```python
from build123d import *

# Parameters (mm, degrees)
L_BASE_DEPTH                                = 12.7
SKETCH3_W                                   = 44.45
SKETCH3_H                                   = 25.4
RECTANGULAR_EXTRUDE_DEPTH                   = 10.5664
SKETCH4_W                                   = 11.1125
SKETCH4_H                                   = 25.4
FORK_EXTRUDE_DEPTH                          = 29.3624
SKETCH6_W                                   = 38.1
SKETCH6_H                                   = 3.175
F_4_EXPANSION_INSERT_RECESSES_1_D           = 3.2639
F_4_EXPANSION_INSERT_RECESSES_1_DEPTH       = 19.05
F_4_EXPANSION_INSERT_RECESSES_1_CBORE_D     = 3.96875
F_4_EXPANSION_INSERT_RECESSES_1_CBORE_DEPTH = 4.7625
F_4_EXPANSION_INSERT_RECESSES_1_TIP         = 0.980574487
F_4_EXPANSION_INSERT_RECESSES_2_D           = 3.2639
F_4_EXPANSION_INSERT_RECESSES_2_DEPTH       = 9.525
F_4_EXPANSION_INSERT_RECESSES_2_CBORE_D     = 3.96875
F_4_EXPANSION_INSERT_RECESSES_2_CBORE_DEPTH = 4.7625
F_4_EXPANSION_INSERT_RECESSES_2_TIP         = 0.980574487


with BuildPart() as part:
    # Sketch1 → L-Base (new body)
    with BuildSketch(Plane(origin=(0, 0, 0), x_dir=(1, 0, 0), z_dir=(0, 1, 0))):
        Polygon((0, 0), (44.45, 0), (44.45, 25.4), (20.066, 25.4), (20.066, 39.116), (0, 39.116), align=None)
    extrude(amount=L_BASE_DEPTH)

    # Sketch3 → Rectangular Extrude (add)
    with BuildSketch(Plane(origin=(0, 12.7, 0), x_dir=(1, 0, 0), z_dir=(0, 1, 0))):
        with Locations((22.225, 12.7)):
            Rectangle(SKETCH3_W, SKETCH3_H)
    extrude(amount=RECTANGULAR_EXTRUDE_DEPTH)

    # Sketch4 → Fork Extrude (add)
    with BuildSketch(Plane(origin=(0, 23.2664, 0), x_dir=(1, 0, 0), z_dir=(0, 1, 0))):
        with Locations((5.55625, 12.7)):
            Rectangle(SKETCH4_W, SKETCH4_H)
        with Locations((38.89375, 12.7)):
            Rectangle(SKETCH4_W, SKETCH4_H)
    extrude(amount=FORK_EXTRUDE_DEPTH)

    # Sketch6 → Shaft Recess (revolve, cut)
    with BuildSketch(Plane(origin=(0, 52.6288, 0), x_dir=(1, 0, 0), z_dir=(0, 1, 0))):
        with Locations((22.225, 11.1125)):
            Rectangle(SKETCH6_W, SKETCH6_H)
    revolve(axis=Axis((0, 52.6288, -12.7), (1, 0, 0)), mode=Mode.SUBTRACT)

    # #4 Expansion Insert Recesses #1
    with Locations(Plane(origin=(0, 52.6288, 0), x_dir=(1, 0, 0), z_dir=(0, 1, 0))):
        with Locations((5.55625, 20.6375), (5.55625, 4.7625), (38.89375, 20.6375), (38.89375, 4.7625)):
            CounterBoreHole(F_4_EXPANSION_INSERT_RECESSES_1_D / 2, F_4_EXPANSION_INSERT_RECESSES_1_CBORE_D / 2, F_4_EXPANSION_INSERT_RECESSES_1_CBORE_DEPTH, depth=F_4_EXPANSION_INSERT_RECESSES_1_DEPTH)
            with Locations((0, 0, -(F_4_EXPANSION_INSERT_RECESSES_1_DEPTH + F_4_EXPANSION_INSERT_RECESSES_1_TIP / 2))):  # 118° drill point
                Cone(0, F_4_EXPANSION_INSERT_RECESSES_1_D / 2, F_4_EXPANSION_INSERT_RECESSES_1_TIP, mode=Mode.SUBTRACT)

    # #4 Expansion Insert Recesses #2
    with Locations(Plane(origin=(0, 0, 0), x_dir=(-1, 0, 0), z_dir=(0, -1, 0))):
        with Locations((-10.033, 10.033), (-29.083, 10.033), (-10.033, 29.083)):
            CounterBoreHole(F_4_EXPANSION_INSERT_RECESSES_2_D / 2, F_4_EXPANSION_INSERT_RECESSES_2_CBORE_D / 2, F_4_EXPANSION_INSERT_RECESSES_2_CBORE_DEPTH, depth=F_4_EXPANSION_INSERT_RECESSES_2_DEPTH)
            with Locations((0, 0, -(F_4_EXPANSION_INSERT_RECESSES_2_DEPTH + F_4_EXPANSION_INSERT_RECESSES_2_TIP / 2))):  # 118° drill point
                Cone(0, F_4_EXPANSION_INSERT_RECESSES_2_D / 2, F_4_EXPANSION_INSERT_RECESSES_2_TIP, mode=Mode.SUBTRACT)


solid = part.part
```
Work out the finished part from the listing and answer in its coordinate system (mm). A direction names the side the tool comes from. Give positions to 0.01 mm unless a question says otherwise; leave off trailing zeros. Loops run counter-clockwise (first coordinate to the right, second up) from the corner with the lowest first, then second, coordinate; pieces in that order, holes last. Notation, with made-up numbers: (-24.75, 48.5) -> (-13.75, 48.5) arc R21 cw to (-13.75, 81.5) -> close; hole circle Ø1 at (-11.75, 7.25). An arc over 180 degrees is marked (long way). One line per question, with ' | ' between items. Start each with the question number.
1) For faces 5 (the face through (41.275, 51, -13)), 6 (the face through (33.338, 38, -13)), 7 (the face through (30.64, 7.18, -10.52)), 8 (the face through (22, 0, -15)), determine the directions among +Z, -Z, +X, -X, +Y, -Y from which every point of the face is accessible in a straight line to the end or side of a thin tool.
2) Determine the mould class of faces 1 (the face through (38.86, 32.77, -20.92)), 2 (the face through (37.362, 49.455, -12.63)), 3 (the face through (22, 20, -25.4)), 4 (the face through (0, 26, -15)) for opening direction X: +X half, -X half, draft (parallel to the pull), parting line (faces both ways), or undercut.
3) Section C-C, the plane x = 34 is taken. Determine the outline of the cut face in (y, z) (3 decimals).
4) Straight lines are drawn through the part: L1, parallel to X at y = 25.5, z = -24; L2, parallel to Z at x = 19, y = 13.5; L3, parallel to Y at x = 32, z = -19.5. For each, find the intervals that lie inside material, in ascending order.
5) Section A-A, the plane y = 44.5 is taken. Determine the outline of the cut face in (x, z).
6) Section B-B, the plane y = 27.5 is taken. Determine the outline of the cut face in (x, z), then the cut area to 3 significant figures.
7) Each of these flat-tipped pins is pushed along its axis until it touches: pin 1 (2 mm diameter, centred on x = 39, z = -4, fed in from +Y); pin 2 (1.2 mm diameter, centred on x = 9.5, z = -28, fed in from -Y); pin 3 (4 mm diameter, centred on x = 10.033, z = -29.083, fed in from +Y). Where does it stop, or does it pass through?
Resolved:
1) face 5: +Y | face 6: +Z, -Z, +Y | face 7: -Y | face 8: +Z, -Z, +X, -X, -Y
2) face 1: undercut | face 2: undercut | face 3: draft | face 4: -X half
3) outline: (0, -25.4) -> (52.629, -25.4) -> (52.629, -15.875) arc R3.175 cw to (52.629, -9.525) -> (52.629, 0) -> (0, 0) -> close
4) L1: 0 to 11.11, 33.34 to 44.45 | L2: -25.4 to 0 | L3: 0 to 23.27
5) outline: (0, -25.4) -> (11.11, -25.4) -> (11.11, 0) -> (0, 0) -> close; (33.34, -25.4) -> (44.45, -25.4) -> (44.45, 0) -> (33.34, 0) -> close; hole circle Ø3.26 at (5.56, -20.64); hole circle Ø3.26 at (5.56, -4.76); hole circle Ø3.26 at (38.89, -20.64); hole circle Ø3.26 at (38.89, -4.76)
6) outline: (0, -25.4) -> (11.11, -25.4) -> (11.11, 0) -> (0, 0) -> close; (33.34, -25.4) -> (44.45, -25.4) -> (44.45, 0) -> (33.34, 0) -> close | area: 565 mm2
7) pin 1: y = 47.87 | pin 2: y = 4.76 | pin 3: y = 12.7
